Verification items for the finished model (mm, model axes). A direction names the side the tool comes from. Give positions to 0.01 mm unless a question says otherwise; leave off trailing zeros. Order: outer loops, then holes, each group sorted by start corner. A loop starts at its lowest first (then second) coordinate and runs counter-clockwise, first axis right, second up. Notation, with made-up numbers: (27, 48) -> (43, 48) arc R24 cw to (43, 77) -> close; hole circle Ø1 at (8, 19). An arc over 180 degrees is marked (long way). One line per question, with ' | ' between items. Start each with the question number.
Q1. Section check D-D on y = 14.25. Record the cut outline in (x, z), plus the area to 3 significant figures.
Q2. Section check A-A on z = 0. Record the cut outline in (x, y).
Q3. Go/stop test with flat-tipped pins: pin 1 (0.6 mm diameter, centred on x = 2, y = 18.5, fed in from -Z); pin 2 (1.5 mm diameter, centred on x = 3.5, y = 12, fed in from -Z); pin 3 (2.5 mm diameter, centred on y = 19, z = 0, fed in from -X); pin 4 (0.5 mm diameter, centred on y = 18.5, z = 0, fed in from -X). Record where each tip stops, or that it passes through.
Q4. Access from +Z, -Z, +X, -X, +Y, -Y to the whole of each face (thin tool, end or side, straight path). Record for faces 1 (the cylindrical face through (-14.04, 18.17, 0.18)), 2 (the cylindrical face through (0.189, 16.647, 11.217)), 3 (the cylindrical face through (-18.146, 18.045, -0.112)).
Q5. Material ranges on probe 1 along Z at (x, y) = (-4.5, 15.25); probe 2 along X at (y, z) = (16.25, 2.25); probe 3 along X at (y, z) = (18.25, -0.75), recorded low to high. Write a range as [from, to].
Q6. Mould release check, pull along X, two halves, no side actions. Record for faces 4 (the cylindrical face through (0.189, 18.045, -12.646)), 5 (the cylindrical face through (-17.718, 12.12, 12.126)), 6 (the cylindrical face through (18.146, 18.045, -0.112)), 7 (the flat face through (14.5, 19, 0)): released by +X, released by -X, zero draft, split by the parting line, or undercut.
Q7. Section check B-B on x = 2. Record the cut outline in (y, z), plus the area to 3 significant figures.
Q8. Section check C-C on y = 11.5. Record the cut outline in (x, z).
from build123d import *

# Parameters (mm, degrees)
SKETCH1_W           = 40
SKETCH1_H           = 29
BOSS_EXTRUDE1_DEPTH = 20
FILLET2_R           = 6.5
SKETCH3_W           = 48.982601016
SKETCH3_H           = 39.309165856
CUT_EXTRUDE1_DEPTH  = 14.5
SHELL1_T            = -2
BOSS_EXTRUDE3_DEPTH = 3
FILLET3_R           = 0.2
SKETCH6_W           = 27
SKETCH6_H           = 15
CUT_EXTRUDE2_DEPTH  = 10.5000001
SKETCH7_R           = 0.85
CUT_EXTRUDE3_DEPTH  = 1.1
CUT_EXTRUDE4_DEPTH  = 1


with BuildPart() as part:
    # Sketch1 → Boss-Extrude1 (new body)
    with BuildSketch(Plane(origin=(0, 0, 0), x_dir=(1, 0, 0), z_dir=(0, 1, 0))):
        Rectangle(SKETCH1_W, SKETCH1_H)
    extrude(amount=BOSS_EXTRUDE1_DEPTH)

    # Fillet2
    fillet2_edges = [part.edges().sort_by_distance(p)[0] for p in [
        (-20, 20, 0),
        (0, 20, 14.5),
        (20, 20, 0),
        (0, 0, 14.5),
        (-20, 0, 0),
        (0, 0, -14.5),
        (20, 0, 0),
        (20, 10, 14.5),
        (-20, 10, 14.5),
        (-20, 10, -14.5),
        (20, 10, -14.5),
        (0, 20, -14.5),
    ]]
    fillet(fillet2_edges, radius=FILLET2_R)

    # Sketch3 → Cut-Extrude1 (cut, through all)
    with BuildSketch(Plane(origin=(0, 13.5, 0), x_dir=(1, 0, 0), z_dir=(0, 1, 0))):
        Rectangle(SKETCH3_W, SKETCH3_H)
    extrude(amount=-CUT_EXTRUDE1_DEPTH, mode=Mode.SUBTRACT)

    # Shell1
    shell1_openings = [part.faces().sort_by_distance(p)[0] for p in [
        (0, 13.5, 0),
    ]]
    offset(amount=SHELL1_T, openings=shell1_openings)

    # Sketch5 → Boss-Extrude3 (add)
    with BuildSketch(Plane.XZ.offset(-13.5)):
        with BuildLine():
            Line((-13.5, 13.9), (-13.5, 13.4))
            ThreePointArc((-13.5, 13.4), (-17.318376618, 11.818376618), (-18.9, 8))
            Line((-18.9, 8), (-19.4, 8))
            ThreePointArc((-19.4, 8), (-17.671930009, 12.171930009), (-13.5, 13.9))
        make_face()
        with BuildLine():
            Line((-19.4, -8), (-18.9, -8))
            ThreePointArc((-18.9, -8), (-17.318376618, -11.818376618), (-13.5, -13.4))
            Line((-13.5, -13.4), (-13.5, -13.9))
            ThreePointArc((-13.5, -13.9), (-17.671930009, -12.171930009), (-19.4, -8))
        make_face()
        with BuildLine():
            Line((13.5, -13.4), (13.5, -13.9))
            ThreePointArc((13.5, -13.9), (17.671930009, -12.171930009), (19.4, -8))
            Line((19.4, -8), (18.9, -8))
            ThreePointArc((18.9, -8), (17.318376618, -11.818376618), (13.5, -13.4))
        make_face()
        with BuildLine():
            Line((19.4, 8), (18.9, 8))
            ThreePointArc((18.9, 8), (17.318376618, 11.818376618), (13.5, 13.4))
            Line((13.5, 13.4), (13.5, 13.9))
            ThreePointArc((13.5, 13.9), (17.671930009, 12.171930009), (19.4, 8))
        make_face()
    extrude(amount=BOSS_EXTRUDE3_DEPTH)

    # Fillet3
    fillet3_edges = [part.edges().sort_by_distance(p)[0] for p in [
        (-17.318376618, 10.5, 11.818376618),
        (-17.671930009, 10.5, 12.171930009),
        (-17.318376618, 10.5, -11.818376618),
        (-17.671930009, 10.5, -12.171930009),
        (17.318376618, 10.5, 11.818376618),
        (17.671930009, 10.5, 12.171930009),
        (17.671930009, 10.5, -12.171930009),
        (-19.15, 10.5, 8),
        (-13.5, 10.5, 13.65),
        (-13.5, 10.5, -13.65),
        (-19.15, 10.5, -8),
        (13.5, 10.5, 13.65),
        (19.15, 10.5, 8),
    ]]
    fillet(fillet3_edges, radius=FILLET3_R)

    # Sketch6 → Cut-Extrude2 (cut, through all)
    with BuildSketch(Plane(origin=(0, 20, 0), x_dir=(1, 0, 0), z_dir=(0, 1, 0))):
        Rectangle(SKETCH6_W, SKETCH6_H)
    extrude(amount=-CUT_EXTRUDE2_DEPTH, mode=Mode.SUBTRACT)

    # Sketch7 → Cut-Extrude3 (cut)
    with BuildSketch(Plane(origin=(-13.5, 0, 0), x_dir=(0, 0, -1), z_dir=(1, 0, 0))):
        with Locations((0, 19)):
            Circle(SKETCH7_R)
    extrude(amount=-CUT_EXTRUDE3_DEPTH, mode=Mode.SUBTRACT)

    # Sketch9 → Cut-Extrude4 (cut)
    with BuildSketch(Plane.ZY.offset(-13.5)):
        with BuildLine():
            Line((0.85, 19), (0.85, 18))
            Line((0.85, 18), (0.85, 17.368151277))
            Line((0.85, 17.368151277), (-0.85, 17.368151277))
            Line((-0.85, 17.368151277), (-0.85, 18))
            Line((-0.85, 18), (-0.85, 19))
            ThreePointArc((-0.85, 19), (0, 19.85), (0.85, 19))
        make_face()
    extrude(amount=-CUT_EXTRUDE4_DEPTH, mode=Mode.SUBTRACT)


solid = part.part
Filled in:
1) outline: (-19.96, -8) arc R6.46 ccw to (-13.5, -14.46) -> (13.5, -14.46) arc R6.46 ccw to (19.96, -8) -> (19.96, 8) arc R6.46 ccw to (13.5, 14.46) -> (-13.5, 14.46) arc R6.46 ccw to (-19.96, 8) -> close; hole (-17.94, -8) arc R4.44 ccw to (-13.5, -12.44) -> (13.5, -12.44) arc R4.44 ccw to (17.94, -8) -> (17.94, 8) arc R4.44 ccw to (13.5, 12.44) -> (-13.5, 12.44) arc R4.44 ccw to (-17.94, 8) -> close | area: 243 mm²
2) outline: (-20, 13.5) -> (-18, 13.5) arc R4.5 cw to (-13.5, 18) -> (-13.5, 18.15) -> (-14.6, 18.15) -> (-14.6, 19.85) -> (-13.5, 19.85) -> (-13.5, 20) arc R6.5 ccw to start; (13.5, 19.85) -> (14.5, 19.85) -> (14.5, 17.89) arc R4.5 cw to (18, 13.5) -> (20, 13.5) arc R6.5 ccw to (13.5, 20) -> close
3) pin 1: z = -12.49 | pin 2: through | pin 3: x = -18.42 | pin 4: x = -17.94
4) face 1: none | face 2: -Y | face 3: +Z, -Z, -X, +Y
5) probe 1: [-14.26, -12.15], [12.15, 14.26] | probe 2: [-19.39, -17.06], [17.06, 19.39] | probe 3: [-17.94, -13.5], [14.5, 17.94]
6) face 4: zero draft | face 5: released by -X | face 6: released by +X | face 7: undercut
7) outline: (13.5, -14.5) arc R6.5 ccw to (20, -8) -> (20, -7.5) -> (18, -7.5) -> (18, -8) arc R4.5 cw to (13.5, -12.5) -> close; (13.5, 12.5) arc R4.5 cw to (18, 8) -> (18, 7.5) -> (20, 7.5) -> (20, 8) arc R6.5 ccw to (13.5, 14.5) -> close | area: 36.6 mm²
8) outline: (-19.4, -8) arc R5.9 ccw to (-13.5, -13.9) -> (-13.5, -13.4) arc R5.4 cw to (-18.9, -8) -> close; (-19.4, 8) -> (-18.9, 8) arc R5.4 cw to (-13.5, 13.4) -> (-13.5, 13.9) arc R5.9 ccw to start; (13.5, -13.9) arc R5.9 ccw to (19.4, -8) -> (18.9, -8) arc R5.4 cw to (13.5, -13.4) -> close; (13.5, 13.4) arc R5.4 cw to (18.9, 8) -> (19.4, 8) arc R5.9 ccw to (13.5, 13.9) -> close
